Read the model definition and answer for the solid it produces. Units are mm, in the model's axes. Give positions to 0.01 mm unless a question says otherwise; leave off trailing zeros. Loops run counter-clockwise (first coordinate to the right, second up) from the corner with the lowest first, then second, coordinate; pieces in that order, holes last. Notation, with made-up numbers: (34.25, 85) -> (44.25, 85) arc R32 cw to (44.25, 119) -> close; hole circle Ø10 at (36.5, 61.25). An arc over 180 degrees is marked (long way). Answer as CSV lines item,"result". Start each with the question number.
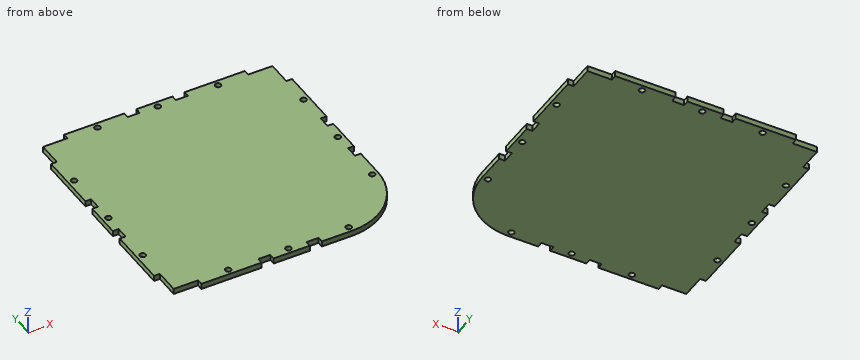
```python
from build123d import *

# Parameters (mm, degrees)
F0_R     = 1.524
F1_DEPTH = 2.9718


with BuildPart() as f1:
    # F0 (on Top) → F1 (new body)
    with BuildSketch(Plane.XY):
        with BuildLine():
            Line((63.5, 15.875), (63.5, 47.625))
            Line((63.5, 47.625), (60.452, 47.625))
            Line((60.452, 47.625), (60.452, 60.452))
            Line((60.452, 60.452), (47.625, 60.452))
            Line((47.625, 60.452), (47.625, 63.5))
            Line((47.625, 63.5), (15.875, 63.5))
            Line((15.875, 63.5), (15.875, 60.452))
            Line((15.875, 60.452), (9.525, 60.452))
            Line((9.525, 60.452), (9.525, 63.5))
            Line((9.525, 63.5), (-9.525, 63.5))
            Line((-9.525, 63.5), (-9.525, 60.452))
            Line((-9.525, 60.452), (-15.875, 60.452))
            Line((-15.875, 60.452), (-15.875, 63.5))
            Line((-15.875, 63.5), (-47.625, 63.5))
            Line((-47.625, 63.5), (-47.625, 60.452))
            Line((-47.625, 60.452), (-60.452, 60.452))
            Line((-60.452, 60.452), (-60.452, 47.625))
            Line((-60.452, 47.625), (-63.5, 47.625))
            Line((-63.5, 47.625), (-63.5, 15.875))
            Line((-63.5, 15.875), (-60.452, 15.875))
            Line((-60.452, 15.875), (-60.452, 9.525))
            Line((-60.452, 9.525), (-63.5, 9.525))
            Line((-63.5, 9.525), (-63.5, -9.525))
            Line((-63.5, -9.525), (-60.452, -9.525))
            Line((-60.452, -9.525), (-60.452, -15.875))
            Line((-60.452, -15.875), (-63.5, -15.875))
            Line((-63.5, -15.875), (-63.5, -47.625))
            Line((-63.5, -47.625), (-60.452, -47.625))
            Line((-60.452, -47.625), (-60.452, -60.452))
            Line((-60.452, -60.452), (-47.625, -60.452))
            Line((-47.625, -60.452), (-47.625, -63.5))
            Line((-47.625, -63.5), (-15.875, -63.5))
            Line((-15.875, -63.5), (-15.875, -60.452))
            Line((-15.875, -60.452), (-9.525, -60.452))
            Line((-9.525, -60.452), (-9.525, -63.5))
            Line((-9.525, -63.5), (9.525, -63.5))
            Line((9.525, -63.5), (9.525, -60.452))
            Line((9.525, -60.452), (15.875, -60.452))
            Line((15.875, -60.452), (15.875, -63.5))
            Line((15.875, -63.5), (31.75, -63.5))
            ThreePointArc((31.75, -63.5), (54.20064, -54.20064), (63.5, -31.75))
            Line((63.5, -31.75), (63.5, -15.875))
            Line((63.5, -15.875), (60.452, -15.875))
            Line((60.452, -15.875), (60.452, -9.525))
            Line((60.452, -9.525), (63.5, -9.525))
            Line((63.5, -9.525), (63.5, 9.525))
            Line((63.5, 9.525), (60.452, 9.525))
            Line((60.452, 9.525), (60.452, 15.875))
            Line((60.452, 15.875), (63.5, 15.875))
        make_face()
        with Locations((-31.75, -60.452)):
            Circle(F0_R, mode=Mode.SUBTRACT)
        with Locations((-60.452, -31.75)):
            Circle(F0_R, mode=Mode.SUBTRACT)
        with Locations((0, -60.452)):
            Circle(F0_R, mode=Mode.SUBTRACT)
        with Locations((31.75, -60.452)):
            Circle(F0_R, mode=Mode.SUBTRACT)
        with Locations((60.452, -31.75)):
            Circle(F0_R, mode=Mode.SUBTRACT)
        with Locations((-60.452, 0)):
            Circle(F0_R, mode=Mode.SUBTRACT)
        with Locations((-60.452, 31.75)):
            Circle(F0_R, mode=Mode.SUBTRACT)
        with Locations((-31.75, 60.452)):
            Circle(F0_R, mode=Mode.SUBTRACT)
        with Locations((60.452, 0)):
            Circle(F0_R, mode=Mode.SUBTRACT)
        with Locations((0, 60.452)):
            Circle(F0_R, mode=Mode.SUBTRACT)
        with Locations((60.452, 31.75)):
            Circle(F0_R, mode=Mode.SUBTRACT)
        with Locations((31.75, 60.452)):
            Circle(F0_R, mode=Mode.SUBTRACT)
    extrude(amount=F1_DEPTH)


solid = f1.part
```
(1) Find section D-D on y = 14. Write down the section's boundary in (x, z), then the cut area to 3 significant figures.
(2) Find section C-C on z = 0.8. Give the number of separate pieces and of enclosed holes in the cut face, then the cut area to 3 significant figures.
(3) Each of these flat-tipped pins is pushed along its axis until it touches: P1, Ø1, axis at x = -6.5, y = -31.5, coming from the -Z side; P2, Ø1.5, axis at y = -62.5, z = 1, coming from the -X side (3 decimals); P3, Ø1.5, axis at y = -44, z = 0.5, coming from the +X side; P4, Ø0.9, axis at y = 12.5, z = 1.5, coming from the +X side. Where does it stop, or does it pass through?
(4) Find the intervals of material crossed by line 1 along Y through (x, z) = (0, 1.9); line 2 along X through (y, z) = (33, 2); line 3 along Y through (x, z) = (-12, 1.2), in increasing order. Write a range as from..to.
(5) Find section A-A on x = -31.75. Write down the section's boundary in (y, z).
Answer block:
1,outline,"(-60.45, 0) -> (60.45, 0) -> (60.45, 2.97) -> (-60.45, 2.97) -> close"
1,area,"359 mm2"
2,separate pieces,"1"
2,enclosed holes,"12"
2,area,"15,400 mm2"
3,P1,"stops at z = 0"
3,P2,"stops at x = -47.625"
3,P3,"stops at x = 61.34"
3,P4,"stops at x = 60.45"
4,line 1,"y = -63.5..-61.98, -58.93..58.93, 61.98..63.5"
4,line 2,"x = -63.5..-61.32, -59.58..59.58, 61.32..63.5"
4,line 3,"y = -60.45..60.45"
5,outline,"(-63.5, 0) -> (-61.98, 0) -> (-61.98, 2.97) -> (-63.5, 2.97) -> close; (-58.93, 0) -> (58.93, 0) -> (58.93, 2.97) -> (-58.93, 2.97) -> close; (61.98, 0) -> (63.5, 0) -> (63.5, 2.97) -> (61.98, 2.97) -> close"
